Part model, mm, in its own coordinate system. A direction names the side the tool comes from. Coordinates: 2 decimals unless noted, no trailing zeros. Order: outer loops, then holes, each group sorted by start corner. A loop starts at its lowest first (then second) coordinate and runs counter-clockwise, first axis right, second up.
```python
from build123d import *

# Parameters (mm, degrees)
BOSS_EXTRUDE2_DEPTH = 7.5
SKETCH6_R           = 3.15
CUT_EXTRUDE1_DEPTH  = 10
SKETCH8_R           = 2.95
BOSS_EXTRUDE3_DEPTH = 2.9


with BuildPart() as part:
    # Sketch1 → Boss-Extrude2 (new, symmetric)
    with BuildSketch(Plane(origin=(0, 0, 0), x_dir=(1, 0, 0), z_dir=(0, 1, 0))):
        Polygon((-0.75, 0), (17.5, 0), (17.5, 19.5), (-0.75, 19.5), (-0.75, 15.5), (12.5, 15.5), (12.5, 5), (6.25, 5), (-0.75, 5), align=None)
    extrude(amount=BOSS_EXTRUDE2_DEPTH, both=True)

    # Sketch6 → Cut-Extrude1 (cut)
    with BuildSketch(Plane.XY):
        with Locations((5.875, 0)):
            Circle(SKETCH6_R)
    extrude(amount=-CUT_EXTRUDE1_DEPTH, mode=Mode.SUBTRACT)

    # Sketch8 → Boss-Extrude3 (add)
    with BuildSketch(Plane(origin=(0, 0, -19.5), x_dir=(-1, 0, 0), z_dir=(0, 0, -1))):
        with Locations(Location((-5.875, 0, 0), (0, 0, 180))):
            Circle(SKETCH8_R)
    extrude(amount=BOSS_EXTRUDE3_DEPTH)


solid = part.part
```
(1) Probe line 1 (Z direction, x = 10.25, y = 5.75); line 2 (X direction, y = -0.5, z = -12.75); line 3 (Z direction, x = 8.25, y = -1.5). List the from-to ranges inside material, lowest first.
(2) Drop flat-ended pins along their axis: pin 1 (8.5 mm diameter, centred on y = -2.5, z = -10, fed in from -X); pin 2 (3 mm diameter, centred on x = 8.5, y = 4.5, fed in from +Z). Give the stop position or say it passes through.
(3) Slice it at D-D, the plane x = 7.75. Give the cut face in (y, z).
(4) Slice it at A-A, the plane x = 11. Give the cut face in (y, z), then the cut area to 3 significant figures.
(5) Pull direction Z, two halves, no side cores. Call faces 1 (the face through (17.5, 0, -10)), 2 (the face through (6, 3.4, -5)), 3 (the face through (10, 0, 0)): +Z half, -Z half, draft (parallel to the pull), parting line (faces both ways), or undercut.
(6) Slice it at C-C, the plane z = -1.5. Give the cut face in (x, y) (3 decimals).
(7) Tool access for faces 4 (the face through (8.785, -1.206, -2.465)), 5 (the face through (6, 0, -15.5)), 6 (the face through (8.689, -0.886, -20.93)), 7 (the face through (14, -7.5, -10)): list every direction of +Z, -Z, +X, -X, +Y, -Y with a clear straight run to the whole face (end or side of a thin tool).
(8) Slice it at B-B, the plane y = 0. Give the cut face in (x, z) (3 decimals), then the cut area to 3 significant figures.
Here are the results:
1. line 1: z = -19.5 to -15.5, -5 to 0
1. line 2: x = 12.5 to 17.5
1. line 3: z = -22.4 to -15.5
2. pin 1: stops at x = 12.5
2. pin 2: stops at z = 0
3. outline: (-7.5, -19.5) - (-2.28, -19.5) - (-2.28, -22.4) - (2.28, -22.4) - (2.28, -19.5) - (7.5, -19.5) - (7.5, -15.5) - (-7.5, -15.5) - close; (-7.5, -5) - (-2.53, -5) - (-2.53, 0) - (-7.5, 0) - close; (2.53, -5) - (7.5, -5) - (7.5, 0) - (2.53, 0) - close
4. outline: (-7.5, -19.5) - (7.5, -19.5) - (7.5, -15.5) - (-7.5, -15.5) - close; (-7.5, -5) - (7.5, -5) - (7.5, 0) - (-7.5, 0) - close
4. area: 135 mm2
5. face 1: draft
5. face 2: undercut
5. face 3: +Z half
6. outline: (-0.75, -7.5) - (17.5, -7.5) - (17.5, 7.5) - (-0.75, 7.5) - close; hole circle Ø6.3 at (5.875, 0)
7. face 4: +Z
7. face 5: -X, +Y, -Y
7. face 6: -Z
7. face 7: +Z, -Z, +X, -X, -Y
8. outline: (-0.75, -19.5) - (2.925, -19.5) - (2.925, -22.4) - (8.825, -22.4) - (8.825, -19.5) - (17.5, -19.5) - (17.5, 0) - (9.025, 0) - (9.025, -5) - (12.5, -5) - (12.5, -15.5) - (-0.75, -15.5) - close; (-0.75, -5) - (2.725, -5) - (2.725, 0) - (-0.75, 0) - close
8. area: 202 mm2
